```python
from build123d import *

# Parameters (mm, degrees)
SKETCH_1_R          = 2.75
EXTRUDE_1_DEPTH     = 3
CUT_EXTRUDE_1_DEPTH = 1.5
SKETCH_3_R          = 1.5
EXTRUDE_2_DEPTH     = 6


with BuildPart() as part:
    # 草图1 → 凸台-拉伸1 (new body)
    with BuildSketch(Plane.XY):
        Circle(SKETCH_1_R)
    extrude(amount=EXTRUDE_1_DEPTH)

    # 草图2 → 切除-拉伸1 (cut)
    with BuildSketch(Plane.XY.offset(3)):
        Polygon((0, -1.443375673), (1.25, -0.721687836), (1.25, 0.721687836), (0, 1.443375673), (-1.25, 0.721687836), (-1.25, -0.721687836), align=None)
    extrude(amount=-CUT_EXTRUDE_1_DEPTH, mode=Mode.SUBTRACT)

    # 草图3 → 凸台-拉伸2 (add)
    with BuildSketch(Plane(origin=(0, 0, 0), x_dir=(-1, 0, 0), z_dir=(0, 0, -1))):
        Circle(SKETCH_3_R)
    extrude(amount=EXTRUDE_2_DEPTH)


solid = part.part
```
Could you check a few things on this model? Use its own coordinates, in mm. A direction names the side the tool comes from. Coordinates: 2 decimals unless noted, no trailing zeros. Write each loop counter-clockwise with the first axis right and the second up, starting at its lowest first coordinate (ties: lowest second). Pieces come first, ordered by that corner, then holes. Notation, with made-up numbers: (77.25, 72) - (84.25, 72) arc R20 ccw to (84.25, 84) - close; hole circle Ø5 at (-19.5, -20.5). An arc over 180 degrees is marked (long way). Use a Markdown table: item, result.
Q1. Please list where these lines run through material, in increasing order: L1, parallel to Z at x = -1.05, y = -2.15; L2, parallel to Z at x = -0.25, y = 0.65; L3, parallel to Y at x = 1, z = 2.
Geometry check:
| item | result |
|---|---|
| L1 | z = 0 to 3 |
| L2 | z = -6 to 1.5 |
| L3 | y = -2.56 to -0.87, 0.87 to 2.56 |
Q2. I'm going to push flat-ended pins straight in: pin 1 Ø2 at (x, z) = (-1, -1.5) entering from -Y; pin 2 Ø2 at (y, z) = (-2, -4) entering from -X; pin 3 Ø1.5 at (x, z) = (-1.5, 1.5) entering from +Y. Where does each tip first touch, or does it pass through?
Geometry check:
| item | result |
|---|---|
| pin 1 | stops at y = -1.5 |
| pin 2 | stops at x = -1.12 |
| pin 3 | stops at y = 2.65 |
Q3. Imagine slicing it at A-A (y = 0). List the corners of the cut face in (x, z) for me, and give its area (4 significant figures).
Geometry check:
| item | result |
|---|---|
| outline | (-2.75, 0) - (-1.5, 0) - (-1.5, -6) - (1.5, -6) - (1.5, 0) - (2.75, 0) - (2.75, 3) - (1.25, 3) - (1.25, 1.5) - (-1.25, 1.5) - (-1.25, 3) - (-2.75, 3) - close |
| area | 30.75 mm2 |
Q4. Thinking about a two-plate mould opening in Y: for faces 1 (the flat face through (0, 0, -6)), 2 (the flat face through (0, 0, 1.5)), 3 (the cylindrical face through (-0.596, -2.685, 1.479)), which applies, +Y half, -Y half, draft (parallel to the pull), parting line (faces both ways), or undercut?
Geometry check:
| item | result |
|---|---|
| face 1 | draft |
| face 2 | undercut |
| face 3 | parting line |
Q5. Imagine slicing it at C-C (z = -3.75). List the corners of the cut face in (x, y) for me, and give its area (3 significant figures).
Geometry check:
| item | result |
|---|---|
| outline | circle Ø3 at (0, 0) |
| area | 7.07 mm2 |
Q6. Which directions (+Z, -Z, +X, -X, +Y, -Y) give clear straight access to the entire face, cutting with the end or side of a thin tool? Please do faces 4 (the flat face through (0.616, -1.088, 2.26)), 5 (the cylindrical face through (1.5, 0.07, -2.96)), 6 (the flat face through (0.6, 1.3, 3)).
Geometry check:
| item | result |
|---|---|
| face 4 | +Z |
| face 5 | -Z |
| face 6 | +Z, +X, -X, +Y, -Y |
Q7. Imagine slicing it at B-B (x = 1.1). List the corners of the cut face in (y, z) for me.
Geometry check:
| item | result |
|---|---|
| outline | (-2.52, 0) - (-1.02, 0) - (-1.02, -6) - (1.02, -6) - (1.02, 0) - (2.52, 0) - (2.52, 3) - (0.81, 3) - (0.81, 1.5) - (-0.81, 1.5) - (-0.81, 3) - (-2.52, 3) - close |
Q8. Imagine slicing it at D-D (z = 0.5). List the corners of the cut face in (x, y) for me.
Geometry check:
| item | result |
|---|---|
| outline | circle Ø5.5 at (0, 0) |
